Drawing for the job (mm, zero at the part's lowest x, y, z). A direction names the side the tool comes from. Round coordinates to 2 decimals unless told otherwise and drop trailing zeros. Loops run counter-clockwise (first coordinate to the right, second up) from the corner with the lowest first, then second, coordinate; pieces in that order, holes last. Notation, with made-up numbers: (69, 15) - (119, 15) arc R22 cw to (119, 52) - close; hole circle Ø4 at (37.25, 36). An arc over 180 degrees is marked (long way). Put each result on its own line as item: value.
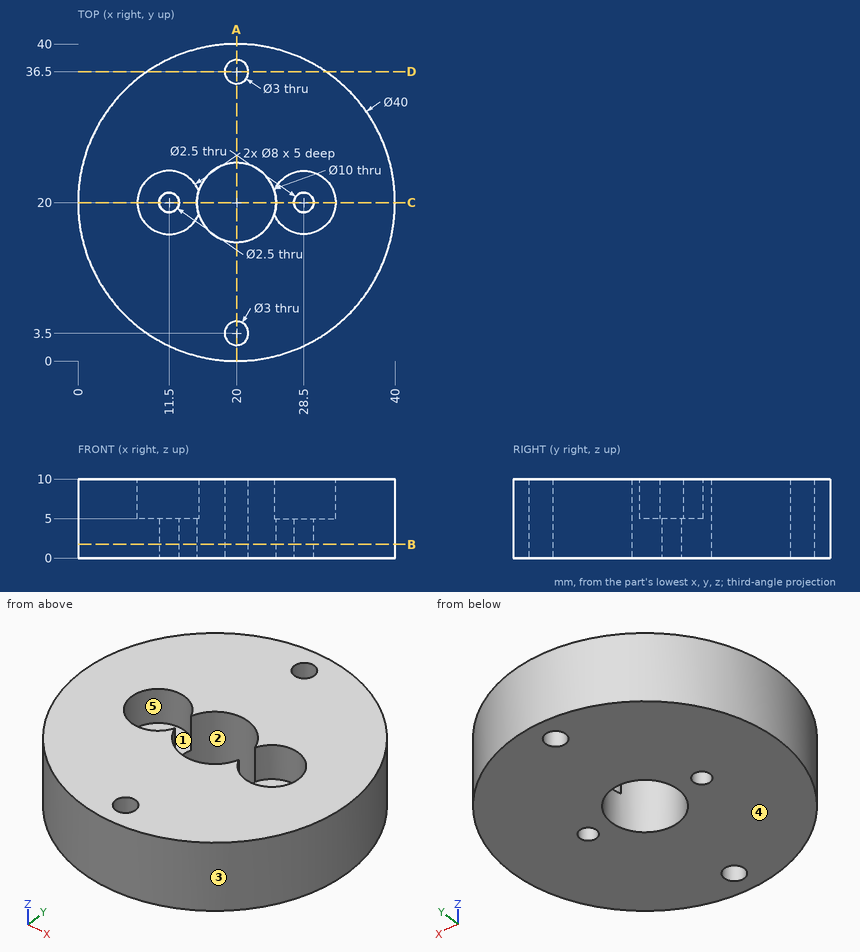
1. Two-plate mould, pull along Y, no slides. Class the marked faces 3, 4 and 5: pulls with the +Y half, pulls with the -Y half, needs draft (parallel to the pull), parting line crosses it, or undercut.
A:
face 3: parting line crosses it
face 4: needs draft
face 5: undercut
2. Band-saw the part on D-D (y = 36.5). List the corners of the cut face in (x, z), plus the area to 3 significant figures.
A:
outline: (8.7, 0) - (18.5, 0) - (18.5, 10) - (8.7, 10) - close; (21.5, 0) - (31.3, 0) - (31.3, 10) - (21.5, 10) - close
area: 196 mm²
3. Band-saw the part on A-A (x = 20). List the corners of the cut face in (y, z), plus the area to 3 significant figures.
A:
outline: (0, 0) - (2, 0) - (2, 10) - (0, 10) - close; (5, 0) - (15, 0) - (15, 10) - (5, 10) - close; (25, 0) - (35, 0) - (35, 10) - (25, 10) - close; (38, 0) - (40, 0) - (40, 10) - (38, 10) - close
area: 240 mm²
4. Band-saw the part on B-B (z = 1.75). List the corners of the cut face in (x, y), plus the area to 3 significant figures.
A:
outline: circle Ø40 at (20, 20); hole circle Ø2.5 at (11.5, 20); hole circle Ø10 at (20, 20); hole circle Ø3 at (20, 3.5); hole circle Ø3 at (20, 36.5); hole circle Ø2.5 at (28.5, 20)
area: 1,150 mm²
5. Band-saw the part on C-C (y = 20). List the corners of the cut face in (x, z), plus the area to 3 significant figures.
A:
outline: (0, 0) - (10.25, 0) - (10.25, 5) - (7.5, 5) - (7.5, 10) - (0, 10) - close; (12.75, 0) - (15, 0) - (15, 5) - (12.75, 5) - close; (25, 0) - (27.25, 0) - (27.25, 5) - (25, 5) - close; (29.75, 0) - (40, 0) - (40, 10) - (32.5, 10) - (32.5, 5) - (29.75, 5) - close
area: 200 mm²
6. Pin check, flat tips, straight feed: P1, Ø9, axis at x = 11.5, y = 20, coming from the +Z side; P2, Ø4, axis at x = 13, y = 21, coming from the +Z side; P3, Ø1.5, axis at x = 11.5, y = 20, coming from the -Z side; P4, Ø1, axis at x = 4.5, z = 9, coming from the +Y side. Stop position of each tip, or through.
A:
P1: stops at z = 10
P2: stops at z = 5
P3: passes through
P4: stops at y = 33.23
7. Tool access for the marked faces 1 and 2: list every direction of +Z, -Z, +X, -X, +Y, -Y with a clear straight run to the whole face (end or side of a thin tool).
A:
face 1: +Z
face 2: +Z, -Z
8. Probe line 1 along Y through (x, z) = (20, 3); line 2 along Y through (x, z) = (19, 8.25); line 3 along Y through (x, z) = (11.5, 1.5). List the from-to ranges inside material, lowest first. Write a range as [from, to].
A:
line 1: y = [0, 2], [5, 15], [25, 35], [38, 40]
line 2: y = [0.03, 2.38], [4.62, 15.1], [24.9, 35.38], [37.62, 39.97]
line 3: y = [1.9, 18.75], [21.25, 38.1]
